For this review, take the finished solid that the model builds, in its own axes (mm). Round coordinates to 2 decimals unless told otherwise and drop trailing zeros. Write each loop counter-clockwise with the first axis right and the second up, starting at its lowest first coordinate (ties: lowest second). Pieces come first, ordered by that corner, then holes. Notation, with made-up numbers: (11, 19.5) -> (31, 19.5) arc R17 ccw to (31, 27.5) -> close; hole circle Ø7 at (39.5, -30). An arc over 180 degrees is marked (long way). Answer in a Markdown table with one row per item. Add a question column.
```python
from build123d import *

# Parameters (mm, degrees)
F0_W     = 17
F0_H     = 4
F1_DEPTH = 5
F3_D     = 2
F4_SIZE2 = 1.9994072094
F4_SIZE  = 1.4
F5_R     = 2
F6_R     = 0.5


with BuildPart() as f1:
    # F0 (on Top) → F1 (new body)
    with BuildSketch(Plane.XY):
        Rectangle(F0_W, F0_H)
    extrude(amount=F1_DEPTH)

    # F3 (through all)
    with Locations(Plane.XY.offset(5)):
        with Locations((6.5, 0)):
            Hole(F3_D / 2)

    # F4
    f4_edges = [f1.edges().sort_by_distance(p)[0] for p in [
        (8.5, -2, 2.5),
        (8.5, 2, 2.5),
    ]]
    f4_side = f1.faces().sort_by_distance((8.5, 0, 2.5))[0]
    chamfer(f4_edges, length=F4_SIZE, length2=F4_SIZE2, reference=f4_side)

    # F5
    f5_edges = [f1.edges().sort_by_distance(p)[0] for p in [
        (6.500593, -2, 2.5),
        (6.500593, 2, 2.5),
    ]]
    fillet(f5_edges, radius=F5_R)

    # F6
    f6_edges = [f1.edges().sort_by_distance(p)[0] for p in [
        (8.5, 0.6, 2.5),
        (8.5, -0.6, 2.5),
    ]]
    fillet(f6_edges, radius=F6_R)


solid = f1.part
```
1. Clearance check with a flat-ended pin moving along its axis: pin 1 Ø3 at (x, z) = (6, 3.5) entering from -Y. State where the tip first meets the part, or that it passes through.
2. For L1, parallel to X at y = 0.5, z = 2.3; L2, parallel to Y at x = 6.5, z = 1; L3, parallel to X at y = 0.7, z = 3.55, list the stretches that pass through material, from the lowest coordinate up. Write a range as [from, to].
3. We need section B-B (z = 2.65). Write out the cut boundary in (x, y), plus the area to 3 significant figures.
4. We need section A-A (y = 0). Write out the cut boundary in (x, z), plus the area to 3 significant figures.
5. The part is to be moulded in two halves that separate along X. For faces 1 (the flat face through (-8.5, 0, 2)), 2 (the cylindrical face through (6.5, -1.9, 2.5)), 3 (the cylindrical face through (7.3, -0.6, 2.5)), 4 (the flat face through (0, 0, 5)), say which applies: pulls with the +X half, pulls with the -X half, needs draft (parallel to the pull), parting line crosses it, or undercut.
6. We need section C-C (x = 6.5). Write out the cut boundary in (y, z).
Response:
| question | item | result |
|---|---|---|
| 1 | pin 1 | y = -2 |
| 2 | L1 | [-8.5, 5.63], [7.37, 8.47] |
| 2 | L2 | [-1.9, -1], [1, 1.9] |
| 2 | L3 | [-8.5, 5.79], [7.21, 8.35] |
| 3 | outline | (-8.5, -2) -> (5.87, -2) arc R2 ccw to (7.02, -1.64) -> (8.29, -0.75) arc R0.5 ccw to (8.5, -0.34) -> (8.5, 0.34) arc R0.5 ccw to (8.29, 0.75) -> (7.02, 1.64) arc R2 ccw to (5.87, 2) -> (-8.5, 2) -> close; hole circle Ø2 at (6.5, 0) |
| 3 | area | 62.0 mm2 |
| 4 | outline | (-8.5, 0) -> (5.5, 0) -> (5.5, 5) -> (-8.5, 5) -> close; (7.5, 0) -> (8.5, 0) -> (8.5, 5) -> (7.5, 5) -> close |
| 4 | area | 75.0 mm2 |
| 5 | face 1 | pulls with the -X half |
| 5 | face 2 | pulls with the +X half |
| 5 | face 3 | undercut |
| 5 | face 4 | needs draft |
| 6 | outline | (-1.9, 0) -> (-1, 0) -> (-1, 5) -> (-1.9, 5) -> close; (1, 0) -> (1.9, 0) -> (1.9, 5) -> (1, 5) -> close |
